CAD build for the part. Positions are in the model's coordinates, mm. Face numbers are marked on the shaded views. Round coordinates to 2 decimals unless told otherwise and drop trailing zeros. Write each loop counter-clockwise with the first axis right and the second up, starting at its lowest first coordinate (ties: lowest second). Pieces come first, ordered by that corner, then holes. Notation, with made-up numbers: (-36, -20.75) -> (21, -20.75) arc R21 cw to (21, -5.75) -> close; hole circle Ø4 at (88.25, -40). An arc over 180 degrees is marked (long way). Answer in a Markdown table with one row per item. Add a question column.
```python
from build123d import *

# Parameters (mm, degrees)
F0_R     = 12.5
F1_DEPTH = 5


with BuildPart() as f1:
    # F0 (on Top) → F1 (new body)
    with BuildSketch(Plane.XY):
        with BuildLine():
            Line((-6.606558, 22.71504), (-7.637189, 23.804902))
            ThreePointArc((-7.637189, 23.804902), (-9.203114, 23.244412), (-10.728305, 22.581042))
            Line((-10.728305, 22.581042), (-10.733541, 21.081051))
            Line((-10.733541, 21.081051), (-12.048001, 20.358421))
            Line((-12.048001, 20.358421), (-13.317291, 21.157735))
            ThreePointArc((-13.317291, 21.157735), (-14.694631, 20.225425), (-16.006933, 19.203596))
            Line((-16.006933, 19.203596), (-15.638972, 17.749428))
            Line((-15.638972, 17.749428), (-16.732425, 16.722607))
            Line((-16.732425, 16.722607), (-18.160619, 17.18115))
            ThreePointArc((-18.160619, 17.18115), (-19.262831, 15.9356), (-20.279786, 14.619518))
            Line((-20.279786, 14.619518), (-19.561748, 13.302543))
            Line((-19.561748, 13.302543), (-20.365488, 12.036051))
            Line((-20.365488, 12.036051), (-21.862848, 12.125011))
            ThreePointArc((-21.862848, 12.125011), (-22.620676, 10.644482), (-23.278385, 9.116841))
            Line((-23.278385, 9.116841), (-22.255388, 8.01981))
            Line((-22.255388, 8.01981), (-22.718913, 6.593226))
            Line((-22.718913, 6.593226), (-24.191354, 6.307012))
            ThreePointArc((-24.191354, 6.307012), (-24.557181, 4.684533), (-24.814318, 3.04132))
            Line((-24.814318, 3.04132), (-23.550639, 2.233164))
            Line((-23.550639, 2.233164), (-23.644825, 0.736123))
            Line((-23.644825, 0.736123), (-24.999828, 0.092721))
            ThreePointArc((-24.999828, 0.092721), (-24.950668, -1.569763), (-24.791076, -3.225299))
            Line((-24.791076, -3.225299), (-23.366118, -3.693801))
            Line((-23.366118, -3.693801), (-23.085046, -5.167232))
            Line((-23.085046, -5.167232), (-24.237471, -6.127397))
            ThreePointArc((-24.237471, -6.127397), (-23.776413, -7.725425), (-23.21012, -9.28926))
            Line((-23.21012, -9.28926), (-21.713417, -9.388671))
            Line((-21.713417, -9.388671), (-21.074748, -10.745911))
            Line((-21.074748, -10.745911), (-21.952185, -11.962507))
            ThreePointArc((-21.952185, -11.962507), (-21.108198, -13.39567), (-20.170786, -14.769543))
            Line((-20.170786, -14.769543), (-18.696383, -14.493616))
            Line((-18.696383, -14.493616), (-17.740247, -15.649386))
            Line((-17.740247, -15.649386), (-18.287562, -17.045969))
            ThreePointArc((-18.287562, -17.045969), (-17.113678, -18.224216), (-15.864048, -19.321801))
            Line((-15.864048, -19.321801), (-14.504586, -18.687874))
            Line((-14.504586, -18.687874), (-13.29106, -19.569551))
            Line((-13.29106, -19.569551), (-13.473864, -21.058371))
            ThreePointArc((-13.473864, -21.058371), (-12.043842, -21.907667), (-10.560513, -22.659999))
            Line((-10.560513, -22.659999), (-9.401412, -21.707904))
            Line((-9.401412, -21.707904), (-8.006748, -22.26009))
            Line((-8.006748, -22.26009), (-7.813554, -23.747597))
            ThreePointArc((-7.813554, -23.747597), (-6.217247, -24.214579), (-4.593422, -24.574387))
            Line((-4.593422, -24.574387), (-3.707514, -23.363946))
            Line((-3.707514, -23.363946), (-2.219342, -23.551946))
            Line((-2.219342, -23.551946), (-1.66229, -24.944675))
            ThreePointArc((-1.66229, -24.944675), (0, -25), (1.66229, -24.944675))
            Line((1.66229, -24.944675), (2.219342, -23.551946))
            Line((2.219342, -23.551946), (3.707514, -23.363946))
            Line((3.707514, -23.363946), (4.593422, -24.574387))
            ThreePointArc((4.593422, -24.574387), (6.217247, -24.214579), (7.813554, -23.747597))
            Line((7.813554, -23.747597), (8.006748, -22.26009))
            Line((8.006748, -22.26009), (9.401412, -21.707904))
            Line((9.401412, -21.707904), (10.560513, -22.659999))
            ThreePointArc((10.560513, -22.659999), (12.043842, -21.907667), (13.473864, -21.058371))
            Line((13.473864, -21.058371), (13.29106, -19.569551))
            Line((13.29106, -19.569551), (14.504586, -18.687874))
            Line((14.504586, -18.687874), (15.864048, -19.321801))
            ThreePointArc((15.864048, -19.321801), (17.113678, -18.224216), (18.287562, -17.045969))
            Line((18.287562, -17.045969), (17.740247, -15.649386))
            Line((17.740247, -15.649386), (18.696383, -14.493616))
            Line((18.696383, -14.493616), (20.170786, -14.769543))
            ThreePointArc((20.170786, -14.769543), (21.108198, -13.39567), (21.952185, -11.962507))
            Line((21.952185, -11.962507), (21.074748, -10.745911))
            Line((21.074748, -10.745911), (21.713417, -9.388671))
            Line((21.713417, -9.388671), (23.21012, -9.28926))
            ThreePointArc((23.21012, -9.28926), (23.776413, -7.725425), (24.237471, -6.127397))
            Line((24.237471, -6.127397), (23.085046, -5.167232))
            Line((23.085046, -5.167232), (23.366118, -3.693801))
            Line((23.366118, -3.693801), (24.791076, -3.225299))
            ThreePointArc((24.791076, -3.225299), (24.950668, -1.569763), (24.999828, 0.092721))
            Line((24.999828, 0.092721), (23.644825, 0.736123))
            Line((23.644825, 0.736123), (23.550639, 2.233164))
            Line((23.550639, 2.233164), (24.814318, 3.04132))
            ThreePointArc((24.814318, 3.04132), (24.557181, 4.684533), (24.191354, 6.307012))
            Line((24.191354, 6.307012), (22.718913, 6.593226))
            Line((22.718913, 6.593226), (22.255388, 8.01981))
            Line((22.255388, 8.01981), (23.278385, 9.116841))
            ThreePointArc((23.278385, 9.116841), (22.620676, 10.644482), (21.862848, 12.125011))
            Line((21.862848, 12.125011), (20.365488, 12.036051))
            Line((20.365488, 12.036051), (19.561748, 13.302543))
            Line((19.561748, 13.302543), (20.279786, 14.619518))
            ThreePointArc((20.279786, 14.619518), (19.262831, 15.9356), (18.160619, 17.18115))
            Line((18.160619, 17.18115), (16.732425, 16.722607))
            Line((16.732425, 16.722607), (15.638972, 17.749428))
            Line((15.638972, 17.749428), (16.006933, 19.203596))
            ThreePointArc((16.006933, 19.203596), (14.694631, 20.225425), (13.317291, 21.157735))
            Line((13.317291, 21.157735), (12.048001, 20.358421))
            Line((12.048001, 20.358421), (10.733541, 21.081051))
            Line((10.733541, 21.081051), (10.728305, 22.581042))
            ThreePointArc((10.728305, 22.581042), (9.203114, 23.244412), (7.637189, 23.804902))
            Line((7.637189, 23.804902), (6.606558, 22.71504))
            Line((6.606558, 22.71504), (5.153683, 23.088074))
            Line((5.153683, 23.088074), (4.775579, 24.539638))
            ThreePointArc((4.775579, 24.539638), (3.133331, 24.802868), (1.477214, 24.956319))
            Line((1.477214, 24.956319), (0.75, 23.644389))
            Line((0.75, 23.644389), (-0.75, 23.644389))
            Line((-0.75, 23.644389), (-1.477214, 24.956319))
            ThreePointArc((-1.477214, 24.956319), (-3.133331, 24.802868), (-4.775579, 24.539638))
            Line((-4.775579, 24.539638), (-5.153683, 23.088074))
            Line((-5.153683, 23.088074), (-6.606558, 22.71504))
        make_face()
        Circle(F0_R, mode=Mode.SUBTRACT)
    extrude(amount=F1_DEPTH)


solid = f1.part
```
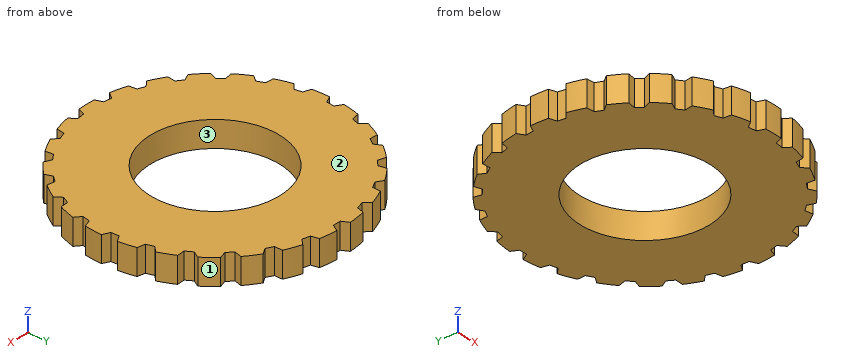
Item 1: Saw through at A-A on x = 0. Give the cut face in (y, z).
Item 2: Saw through at B-B on y = 5. Give the cut face in (x, z), then the cut area to 3 significant figures.
Item 3: Drill centre lines: probe 1 along Y at (x, z) = (0, 1.05); probe 2 along Y at (x, z) = (-3, 3.2); probe 3 along X at (y, z) = (10, 4). Where is each one in solid material? Low to high.
Item 4: Pin check, flat tips, straight feed: pin 1 (1 mm diameter, centred on y = -16.5, z = 3, fed in from -X); pin 2 (22.5 mm diameter, centred on x = 0, y = 0, fed in from +Z); pin 3 (8 mm diameter, centred on x = 10.5, y = 17, fed in from -Z). Stop position of each tip, or through.
Item 5: Two-plate mould, pull along X, no slides. Class the marked faces 1, 2 and 3: +X half, -X half, draft (parallel to the pull), parting line (faces both ways), or undercut.
Recorded:
| question | item | result |
|---|---|---|
| 1 | outline | (-25, 0) -> (-12.5, 0) -> (-12.5, 5) -> (-25, 5) -> close; (12.5, 0) -> (23.64, 0) -> (23.64, 5) -> (12.5, 5) -> close |
| 2 | outline | (-24.49, 0) -> (-11.46, 0) -> (-11.46, 5) -> (-24.49, 5) -> close; (11.46, 0) -> (24.49, 0) -> (24.49, 5) -> (11.46, 5) -> close |
| 2 | area | 130 mm2 |
| 3 | probe 1 | -25 to -12.5, 12.5 to 23.64 |
| 3 | probe 2 | -23.45 to -12.13, 12.13 to 24.82 |
| 3 | probe 3 | -22.91 to -7.5, 7.5 to 22.91 |
| 4 | pin 1 | x = -18.27 |
| 4 | pin 2 | through |
| 4 | pin 3 | z = 0 |
| 5 | face 1 | +X half |
| 5 | face 2 | draft |
| 5 | face 3 | undercut |
